from build123d import *

# Parameters (mm, degrees)
SKETCH_1_W          = 45
SKETCH_1_H          = 43
SKETCH_1_W_2        = 8
SKETCH_1_H_2        = 3
SKETCH_1_W_3        = 3
SKETCH_1_H_3        = 15
EXTRUDE_1_DEPTH     = 3
SKETCH_2_W          = 10
SKETCH_2_H          = 15
CUT_EXTRUDE_1_DEPTH = 10


with BuildPart() as part:
    # 草图1 → 凸台-拉伸1 (new body)
    with BuildSketch(Plane.XY):
        Rectangle(SKETCH_1_W, SKETCH_1_H)
        with Locations((-13.5, 23)):
            Rectangle(SKETCH_1_W_2, SKETCH_1_H_2)
        with Locations((13.5, 23)):
            Rectangle(SKETCH_1_W_2, SKETCH_1_H_2)
        with Locations((-24, 0)):
            Rectangle(SKETCH_1_W_3, SKETCH_1_H_3)
        with Locations((24, 0)):
            Rectangle(SKETCH_1_W_3, SKETCH_1_H_3)
        with Locations((-13.5, -23)):
            Rectangle(SKETCH_1_W_2, SKETCH_1_H_2)
        with Locations((13.5, -23)):
            Rectangle(SKETCH_1_W_2, SKETCH_1_H_2)
    extrude(amount=EXTRUDE_1_DEPTH)

    # 草图2 → 切除-拉伸1 (cut)
    with BuildSketch(Plane.XY.offset(3)):
        with Locations((0, -14)):
            Rectangle(SKETCH_2_W, SKETCH_2_H)
    extrude(amount=-CUT_EXTRUDE_1_DEPTH, mode=Mode.SUBTRACT)


solid = part.part
Could you check a few things on this model? Use its own coordinates, in mm. A direction names the side the tool comes from. Coordinates: 2 decimals unless noted, no trailing zeros. Order: outer loops, then holes, each group sorted by start corner. A loop starts at its lowest first (then second) coordinate and runs counter-clockwise, first axis right, second up.
Q1. Suppose I cut it at A-A on y = -17. Please give me the cut outline in (x, z), and give its area (3 significant figures).
Q2. Suppose I cut it at C-C on x = 6. Please give me the cut outline in (y, z).
Q3. Which directions (+Z, -Z, +X, -X, +Y, -Y) give clear straight access to the entire face, cutting with the end or side of a thin tool? Please do faces 1 (the flat face through (0, 21.5, 1)), 2 (the flat face through (0, -6.5, 2)), 3 (the flat face through (-24, 7.5, 1)), 4 (the flat face through (22.5, 14, 1)), 5 (the flat face through (-22.5, -15, 1)).
Q4. Thinking about a two-plate mould opening in X: for faces 6 (the flat face through (20, 21.5, 1)), 7 (the flat face through (9.5, 23, 1)), 8 (the flat face through (-22.5, 14, 1)), which applies, released by +X, released by -X, zero draft, split by the parting line, or undercut?
Q5. Suppose I cut it at D-D on y = 10.5. Please give me the cut outline in (x, z), and give its area (3 significant figures).
Q6. Will these pins go through, and if not, where does the flat tip stop? pin 1 (0.9 mm diameter, centred on x = 24, z = 2, fed in from +Y); pin 2 (0.9 mm diameter, centred on x = -8, z = 2, fed in from -Y); pin 3 (0.9 mm diameter, centred on y = -23.5, z = 2, fed in from -X).
Q7. Please list where these lines run through material, in increasing order: L1, parallel to X at y = -9.5, z = 2.85; L2, parallel to Y at x = -19, z = 1.7; L3, parallel to X at y = 18, z = 0.45.
Answer:
1. outline: (-22.5, 0) - (-5, 0) - (-5, 3) - (-22.5, 3) - close; (5, 0) - (22.5, 0) - (22.5, 3) - (5, 3) - close
1. area: 105 mm2
2. outline: (-21.5, 0) - (21.5, 0) - (21.5, 3) - (-21.5, 3) - close
3. face 1: +Z, -Z, +Y
3. face 2: +Z, -Z, -Y
3. face 3: +Z, -Z, -X, +Y
3. face 4: +Z, -Z, +X, +Y
3. face 5: +Z, -Z, -X, -Y
4. face 6: zero draft
4. face 7: undercut
4. face 8: released by -X
5. outline: (-22.5, 0) - (22.5, 0) - (22.5, 3) - (-22.5, 3) - close
5. area: 135 mm2
6. pin 1: stops at y = 7.5
6. pin 2: stops at y = -21.5
6. pin 3: stops at x = -17.5
7. L1: x = -22.5 to -5, 5 to 22.5
7. L2: y = -21.5 to 21.5
7. L3: x = -22.5 to 22.5
